Source: CAD feature listing. Evaluate the final solid. Frame: model axes, mm. A direction names the side the tool comes from. Round coordinates to 2 decimals unless told otherwise and drop trailing zeros. Loops run counter-clockwise (first coordinate to the right, second up) from the corner with the lowest first, then second, coordinate; pieces in that order, holes last. Notation, with made-up numbers: (-27, -6.75) -> (-17, -6.75) arc R18 cw to (-17, 0.25) -> close; hole circle Ø4 at (10, 76). An arc over 180 degrees is marked (long way). Put each result on its own line as item: value. Start each with the question number.
1. Material intervals for L1, parallel to Y at x = 10.75, z = 4; L2, parallel to Y at x = 15, z = 6.5; L3, parallel to X at y = -14, z = 2.25, sorted ascending.
2. Cut plane D-D (y = -7). Return the cut outline in (x, z), then the cut area to 3 significant figures.
3. Cut plane B-B (y = 13.5). Return the cut outline in (x, z).
4. Cut plane A-A (x = 3.25). Return the cut outline in (y, z), then the cut area to 3 significant figures.
5. Draft query along Y for faces 1 (the flat face through (1, -2, 8.89)), 2 (the flat face through (11, -24.13, 5)), 3 (the flat face through (15, -10.287, 4)). Return one class per face: pulls with the +Y half, pulls with the -Y half, needs draft (parallel to the pull), parting line crosses it, or undercut.
6. Cut plane C-C (z = 4.5). Return the cut outline in (x, y).
7. Set-up query: faces 4 (the flat face through (19.987, 0, 6)), 5 (the flat face through (0, 0, 4)). Return all of +Z, -Z, +X, -X, +Y, -Y with unobstructed straight access to the full face (end or side cutting, diameter ignored); none if empty.
```python
from build123d import *

# Parameters (mm, degrees)
F0_W     = 21.336
F0_H     = 8.89
F1_DEPTH = 24.13
F3_DEPTH = 21.59
F4_W     = 13.57103
F4_H     = 8.926946
F5_DEPTH = 10.287


with BuildPart() as f1:
    # F0 (on Front) → F1 (new body, symmetric)
    with BuildSketch(Plane.XZ):
        with Locations((10.668, 4.445)):
            Rectangle(F0_W, F0_H)
    extrude(amount=F1_DEPTH, both=True)

    # F2 (on Front) → F3 (cut, symmetric)
    with BuildSketch(Plane.XZ):
        Polygon((19.987223, 8.89), (1.27, 8.89), (3.876193, 1.729542), (6.416193, 1.729542), (6.416193, 2.654027), (19.987223, 7.593478), align=None)
    extrude(amount=F3_DEPTH, both=True, mode=Mode.SUBTRACT)

    # F4 (on Front) → F5 (cut, symmetric)
    with BuildSketch(Plane.XZ):
        with Locations((13.201708, 6.193015)):
            Rectangle(F4_W, F4_H)
    extrude(amount=F5_DEPTH, both=True, mode=Mode.SUBTRACT)


solid = f1.part
```
Solution:
1. L1: y = -24.13 to -10.29, 10.29 to 24.13
1. L2: y = -24.13 to -21.59, 21.59 to 24.13
1. L3: x = 0 to 3.69, 6.42 to 21.34
2. outline: (0, 0) -> (21.34, 0) -> (21.34, 8.89) -> (19.99, 8.89) -> (19.99, 1.73) -> (3.88, 1.73) -> (1.27, 8.89) -> (0, 8.89) -> close
2. area: 65.0 mm^2
3. outline: (0, 0) -> (21.34, 0) -> (21.34, 8.89) -> (19.99, 8.89) -> (19.99, 7.59) -> (6.42, 2.65) -> (6.42, 1.73) -> (3.88, 1.73) -> (1.27, 8.89) -> (0, 8.89) -> close
4. outline: (-24.13, 0) -> (24.13, 0) -> (24.13, 8.89) -> (21.59, 8.89) -> (21.59, 3.45) -> (-21.59, 3.45) -> (-21.59, 8.89) -> (-24.13, 8.89) -> close
4. area: 194 mm^2
5. face 1: needs draft
5. face 2: pulls with the -Y half
5. face 3: undercut
6. outline: (0, -24.13) -> (21.34, -24.13) -> (21.34, 24.13) -> (0, 24.13) -> close; hole (2.87, -21.59) -> (11.49, -21.59) -> (11.49, -10.29) -> (19.99, -10.29) -> (19.99, 10.29) -> (11.49, 10.29) -> (11.49, 21.59) -> (2.87, 21.59) -> close
7. face 4: +Z
7. face 5: +Z, -Z, -X, +Y, -Y
